Source: CAD feature listing. Evaluate the final solid. Frame: model axes, mm. Coordinates: 2 decimals unless noted, no trailing zeros. Loops run counter-clockwise (first coordinate to the right, second up) from the corner with the lowest first, then second, coordinate; pieces in that order, holes last.
from build123d import *

# Parameters (mm, degrees)
SKETCH1_W           = 180
SKETCH1_H           = 180
BOSS_EXTRUDE1_DEPTH = 2
SKETCH2_R           = 1.5
SKETCH2_W           = 15
SKETCH2_H           = 75
SKETCH2_W_2         = 140
SKETCH2_H_2         = 3
CUT_EXTRUDE1_DEPTH  = 2
SKETCH3_R           = 1.5
CUT_EXTRUDE2_DEPTH  = 3


with BuildPart() as part:
    # Sketch1 → Boss-Extrude1 (new body)
    with BuildSketch(Plane(origin=(0, 0, 0), x_dir=(1, 0, 0), z_dir=(0, 1, 0))):
        Rectangle(SKETCH1_W, SKETCH1_H)
    extrude(amount=BOSS_EXTRUDE1_DEPTH)

    # Sketch2 → Cut-Extrude1 (cut)
    with BuildSketch(Plane(origin=(0, 2, 0), x_dir=(1, 0, 0), z_dir=(0, 1, 0))):
        with Locations(Location((-80, 38, 0), (0, 0, 270))):
            Circle(SKETCH2_R)
        with Locations(Location((-80, -82, 0), (0, 0, 270))):
            Circle(SKETCH2_R)
        with Locations(Location((80, -82, 0), (0, 0, 90))):
            Circle(SKETCH2_R)
        with Locations(Location((80, 38, 0), (0, 0, 90))):
            Circle(SKETCH2_R)
        with Locations(Location((-80, 80, 0), (0, 0, 270))):
            Circle(SKETCH2_R)
        with Locations(Location((-80, 50, 0), (0, 0, 270))):
            Circle(SKETCH2_R)
        with Locations(Location((80, 50, 0), (0, 0, 90))):
            Circle(SKETCH2_R)
        with Locations(Location((80, 80, 0), (0, 0, 90))):
            Circle(SKETCH2_R)
        with Locations((-82.5, -37.5)):
            Rectangle(SKETCH2_W, SKETCH2_H)
        with Locations((82.5, -37.5)):
            Rectangle(SKETCH2_W, SKETCH2_H)
        with Locations((0, 81.5)):
            Rectangle(SKETCH2_W_2, SKETCH2_H_2)
    extrude(amount=-CUT_EXTRUDE1_DEPTH, mode=Mode.SUBTRACT)

    # Sketch3 → Cut-Extrude2 (cut)
    with BuildSketch(Plane(origin=(0, 2, 0), x_dir=(1, 0, 0), z_dir=(0, 1, 0))):
        with Locations(Location((-50, -23.75, 0), (0, 0, 270))):
            Circle(SKETCH3_R)
        with Locations(Location((-50, -51.25, 0), (0, 0, 270))):
            Circle(SKETCH3_R)
        with Locations(Location((-25, -23.75, 0), (0, 0, 270))):
            Circle(SKETCH3_R)
        with Locations(Location((-25, -51.25, 0), (0, 0, 270))):
            Circle(SKETCH3_R)
        with Locations(Location((25, -23.75, 0), (0, 0, 270))):
            Circle(SKETCH3_R)
        with Locations(Location((50, -23.75, 0), (0, 0, 270))):
            Circle(SKETCH3_R)
        with Locations(Location((25, -51.25, 0), (0, 0, 270))):
            Circle(SKETCH3_R)
        with Locations(Location((50, -51.25, 0), (0, 0, 270))):
            Circle(SKETCH3_R)
    extrude(amount=-CUT_EXTRUDE2_DEPTH, mode=Mode.SUBTRACT)


solid = part.part
Q1. Section B-B, the plane x = -13.5. Return the cut outline in (y, z).
Q2. Contact query for a flat-ended pin moving along its axis: pin 1 Ø1.8 at (x, z) = (-25, 23.75) entering from +Y. Output: stop coordinate, or through.
Q3. Section C-C, the plane z = 5. Return the cut outline in (x, y), plus the area to 3 significant figures.
Q4. Section A-A, the plane y = 1.1. Count the separate pieces of the cut face and the enclosed holes in it, plus the area to 3 significant figures.
Q5. Line query: line 1 along Z through (x, y) = (80, 1.7); line 2 along X through (y, z) = (0.55, -38); line 3 along X through (y, z) = (1.35, 51.25). Output: solid intervals per line, ascending.
Derived:
1. outline: (0, -90) - (2, -90) - (2, -83) - (0, -83) - close; (0, -80) - (2, -80) - (2, 90) - (0, 90) - close
2. pin 1: passes through
3. outline: (-75, 0) - (75, 0) - (75, 2) - (-75, 2) - close
3. area: 300 mm2
4. separate pieces: 1
4. enclosed holes: 17
4. area: 29,600 mm2
5. line 1: z = -90 to -81.5, -78.5 to -51.5, -48.5 to -39.5, -36.5 to 0, 75 to 80.5, 83.5 to 90
5. line 2: x = -90 to -81.5, -78.5 to 78.5, 81.5 to 90
5. line 3: x = -75 to -51.5, -48.5 to -26.5, -23.5 to 23.5, 26.5 to 48.5, 51.5 to 75
